```python
from build123d import *

# Parameters (mm, degrees)
F0_W     = 152.6974141598
F0_H     = 68.2531446218
F1_DEPTH = 25.4
F2_DEPTH = 25.4
F3_T     = -2.54
F4_DEPTH = 25.4
F5_R     = 11.1655265509
F5_R_2   = 11.2527895093
F5_R_3   = 12.2950319863
F5_R_4   = 13.1342738177
F5_R_5   = 12.1678107689
F5_R_6   = 11.5067470657
F5_R_7   = 11.4719197335
F5_R_8   = 11.2409300987
F6_DEPTH = 11.901790014
F7_DEPTH = 9.59548
F8_R     = 17.8222476658
F8_R_2   = 19.5893706017
F9_DEPTH = 22.97085


with BuildPart() as f1:
    # F0 (on Front) → F1 (new body)
    with BuildSketch(Plane.XZ):
        Rectangle(F0_W, F0_H)
    extrude(amount=F1_DEPTH)

    # F2 (add): a face of the model
    f2_faces = [f1.faces().sort_by_distance(p)[0] for p in [
        (0, -25.4, 0),
    ]]
    extrude(f2_faces, amount=F2_DEPTH)

    # F3
    f3_openings = [f1.faces().sort_by_distance(p)[0] for p in [
        (0, -50.8, 0),
    ]]
    offset(amount=F3_T, openings=f3_openings)

    # F4 (add): a face of the model
    f4_faces = [f1.faces().sort_by_distance(p)[0] for p in [
        (0, -2.54, 0),
    ]]
    extrude(f4_faces, amount=F4_DEPTH)

    # F5 (on face) → F6 (join)
    with BuildSketch(Plane(origin=(0, 0, 0), x_dir=(-1, 0, 0), z_dir=(0, 1, 0))):
        with Locations((60.2360665798, -18.3391999453)):
            Circle(F5_R)
        with Locations((23.5576685518, -18.6373982579)):
            Circle(F5_R_2)
        with Locations((-16.9973094016, -18.3391999453)):
            Circle(F5_R_3)
        with Locations((-56.0612902045, -18.6373982579)):
            Circle(F5_R_4)
        with Locations((-57.8504800797, 17.7428014576)):
            Circle(F5_R_5)
        with Locations((-17.8919043392, 17.4446031451)):
            Circle(F5_R_6)
        with Locations((23.2594702393, 16.8482083827)):
            Circle(F5_R_7)
        with Locations((59.9378682673, 17.1464048326)):
            Circle(F5_R_8)
    extrude(amount=F6_DEPTH)

    # F5 (on face) → F7 (join)
    with BuildSketch(Plane(origin=(0, 0, 0), x_dir=(-1, 0, 0), z_dir=(0, 1, 0))):
        with Locations((60.2360665798, -18.3391999453)):
            Circle(F5_R)
        with Locations((23.5576685518, -18.6373982579)):
            Circle(F5_R_2)
        with Locations((59.9378682673, 17.1464048326)):
            Circle(F5_R_8)
        with Locations((23.2594702393, 16.8482083827)):
            Circle(F5_R_7)
        with Locations((-16.9973094016, -18.3391999453)):
            Circle(F5_R_3)
        with Locations((-56.0612902045, -18.6373982579)):
            Circle(F5_R_4)
        with Locations((-17.8919043392, 17.4446031451)):
            Circle(F5_R_6)
        with Locations((-57.8504800797, 17.7428014576)):
            Circle(F5_R_5)
    extrude(amount=F7_DEPTH)

    # F8 (on face) → F9 (join)
    with BuildSketch(Plane.XZ.offset(27.94)):
        with Locations((-37.5465936959, 0)):
            Circle(F8_R)
        with Locations((37.8445833921, 0)):
            Circle(F8_R_2)
    extrude(amount=F9_DEPTH)


solid = f1.part
```
Here's how the part is built. I have some questions about the finished solid (model axes, mm). A direction names the side the tool comes from. Coordinates: 2 decimals unless noted, no trailing zeros. Order: outer loops, then holes, each group sorted by start corner. A loop starts at its lowest first (then second) coordinate and runs counter-clockwise, first axis right, second up. Notation, with made-up numbers: (87, 35) -> (143, 35) arc R32 ccw to (143, 61) -> close; hole circle Ø4 at (30, 57.25). An arc over 180 degrees is marked (long way). Return JSON: item names as keys, results as strings.
1) If we section it at A-A on y = -46.5: List the corners of the cut face in (x, z) for me, plus the area to 3 significant figures.
Conclusion:
{"outline": "(-76.35, -34.13) -> (76.35, -34.13) -> (76.35, 34.13) -> (-76.35, 34.13) -> close; circle Ø35.64 at (-37.55, 0); circle Ø39.18 at (37.84, 0); hole (-73.81, -31.59) -> (73.81, -31.59) -> (73.81, 31.59) -> (-73.81, 31.59) -> close", "area": "3,300 mm²"}
2) On a 3-axis mill with a long thin cutter (end or side, diameter ignored), from which of +Z, -Z, +X, -X, +Y, -Y can I reach the whole of each face in a straight line? I mean faces 4 (the flat face through (-1, -39, -31.587)), 5 (the flat face through (18, 11.902, 18)), 6 (the cylindrical face through (66.484, 5.868, -26.629)). Say none if no direction works.
Conclusion:
{"face 4": "-Y", "face 5": "+Z, -Z, +X, -X, +Y", "face 6": "+Y"}
3) If we section it at C-C on x = 53: List the corners of the cut face in (y, z) for me.
Conclusion:
{"outline": "(-50.91, -12.41) -> (-27.94, -12.41) -> (-27.94, -31.59) -> (-50.8, -31.59) -> (-50.8, -34.13) -> (0, -34.13) -> (0, -31.41) -> (11.9, -31.41) -> (11.9, -5.86) -> (0, -5.86) -> (0, 6.58) -> (11.9, 6.58) -> (11.9, 28.9) -> (0, 28.9) -> (0, 34.13) -> (-50.8, 34.13) -> (-50.8, 31.59) -> (-27.94, 31.59) -> (-27.94, 12.41) -> (-50.91, 12.41) -> close"}
4) I'm going to push flat-ended pins straight in: P1, Ø2, axis at x = 13.5, z = -3, coming from the +Y side; P2, Ø1, axis at x = -14, z = 14.5, coming from the -Y side. Where does each tip first touch, or does it pass through?
Conclusion:
{"P1": "stops at y = 0", "P2": "stops at y = -27.94"}
5) Thinking about a two-plate mould opening in Z: for faces 1 (the cylindrical face through (22.3, -39.26, -11.92)), 2 (the flat face through (-1, -25, 34.127)), 3 (the flat face through (-23, 11.902, -18)), which applies, +Z half, -Z half, draft (parallel to the pull), parting line (faces both ways), or undercut?
Conclusion:
{"face 1": "undercut", "face 2": "+Z half", "face 3": "draft"}
6) If I drill on probe 1 along X at (y, z) = (-47, -31); probe 2 along X at (y, z) = (-28, 15.5); probe 3 along Z at (x, y) = (60.5, -46), over which ranges is the centre line in solid material (lowest first)?
Conclusion:
{"probe 1": "x = -76.35 to -73.81, 73.81 to 76.35", "probe 2": "x = -76.35 to -73.81, -46.34 to -28.75, 25.87 to 49.82, 73.81 to 76.35", "probe 3": "z = -34.13 to -31.59, 31.59 to 34.13"}
7) If we section it at B-B on z = 0: List the corners of the cut face in (x, y) for me.
Conclusion:
{"outline": "(-76.35, -50.8) -> (-73.81, -50.8) -> (-73.81, -27.94) -> (-55.37, -27.94) -> (-55.37, -50.91) -> (-19.72, -50.91) -> (-19.72, -27.94) -> (18.26, -27.94) -> (18.26, -50.91) -> (57.43, -50.91) -> (57.43, -27.94) -> (73.81, -27.94) -> (73.81, -50.8) -> (76.35, -50.8) -> (76.35, 0) -> (-76.35, 0) -> close"}
